Here's how the part is built. I have some questions about the finished solid (model axes, mm). A direction names the side the tool comes from. Coordinates: 2 decimals unless noted, no trailing zeros. Loops run counter-clockwise (first coordinate to the right, second up) from the corner with the lowest first, then second, coordinate; pieces in that order, holes last. Notation, with made-up numbers: M 81,77.5 L 100,77.5 A17 ccw 100,85.5 Z; hole C 71,39 d9. An arc over 180 degrees is marked long. Use CSV: the item, a comma, the result in double quotes. Start each with the question number.
Q1. If we mould it in two halves opening along Z, with no side actions, what happens to faces 3 (the cylindrical face through (103.673, -1.721, 9.021)), 4 (the flat face through (104, 14, 0)), 5 (the cylindrical face through (100.94, 0.8, 5.94))? For each: +Z half, -Z half, draft (parallel to the pull), parting line (faces both ways), or undercut.
Q2. If we section it at C-C (y = 22): Please give me the cut outline in (x, z).
Q3. If we section it at B-B (x = 98.5): Please give me the cut outline in (y, z).
Q4. For pin 1 Ø1.7 at (x, z) = (102.338, 6) entering from +Y, with a flat end and sliding along its axis, tell me the tip position at first contact or that it passes through.
Q5. If we section it at A-A (z = 4): Please give me the cut outline in (x, y), and give its area (3 significant figures).
Q6. Which directions (+Z, -Z, +X, -X, +Y, -Y) give clear straight access to the entire face, cutting with the end or side of a thin tool? Please do faces 1 (the flat face through (101, 10.1, 5)), 2 (the cylindrical face through (100.94, -1.36, 2.29)).
Q7. Please list where these lines run through material, in increasing order: probe 1 along Y at (x, z) = (98.5, 1.25); probe 2 along X at (y, z) = (-0.4, 6); probe 3 along Y at (x, z) = (101.5, 4). Write a range as [from, to].
Autodesk Inventor part; units mm, degrees
ref_plane "YZ Plane" through (0, 0, 0) normal (1, 0, 0) x (0, 1, 0)
ref_plane "XZ Plane" through (0, 0, 0) normal (0, 1, 0) x (-1, 0, 0)
ref_plane "XY Plane" through (0, 0, 0) normal (0, 0, 1) x (1, 0, 0)
ref_plane "Arbeitsebene1" through (0, 0, 0) normal (0, 0, 1) x (1, 0, 0)
sketch "Skizze1" plane through (0, 0, 0) normal (0, 0, 1) x (1, 0, 0)
  line L0 (-118.5, -74.5) -> (-118.5, 74.5)
  arc A0 (-118.5, -74.5) -> (-103.5, -89.5) centre (-103.5, -74.5) ccw
  line L1 (56.1, -89.5) -> (-103.5, -89.5)
  line L2 (56.1, -83) -> (56.1, -89.5)
  arc A1 (71.1, -68) -> (56.1, -83) centre (71.1, -83) ccw
  line L3 (80.5, -68) -> (71.1, -68)
  arc A2 (95.5, -83) -> (80.5, -68) centre (80.5, -83) ccw
  line L4 (95.5, -89.5) -> (95.5, -83)
  line L5 (103.5, -89.5) -> (95.5, -89.5)
  arc A3 (103.5, -89.5) -> (118.5, -74.5) centre (103.5, -74.5) ccw
  line L6 (118.5, 74.5) -> (118.5, -74.5)
  arc A4 (118.5, 74.5) -> (103.5, 89.5) centre (103.5, 74.5) ccw
  line L7 (-103.5, 89.5) -> (103.5, 89.5)
  arc A5 (-103.5, 89.5) -> (-118.5, 74.5) centre (-103.5, 74.5) ccw
  circle A6 centre (-58.5, 18.7) radius 1.4
  circle A7 centre (-58.5, 36.552) radius 1.4
  circle A8 centre (57.5, 20.252) radius 1.4
  circle A9 centre (57.5, 35) radius 1.4
  circle A10 centre (-58.5, 8.7) radius 1.4
  circle A11 centre (-58.5, -9.152) radius 1.4
  circle A12 centre (57.5, 7.148) radius 1.4
  circle A13 centre (57.5, -7.6) radius 1.4
  circle A14 centre (103.5, 74.5) radius 1.4
  circle A15 centre (103.5, -74.5) radius 1.4
  circle A16 centre (-103.5, -74.5) radius 1.4
  circle A17 centre (-103.5, 74.5) radius 1.4
  line L8 (20.9567, 0.5738) -> (-20.9567, 0.5738)
  line L9 (-20.9567, 0.5738) -> (-20.9567, 30.6837)
  line L10 (-20.9567, 30.6837) -> (20.9567, 30.6837)
  line L11 (20.9567, 30.6837) -> (20.9567, 0.5738)
  circle A18 centre (73.1917, -22.4328) radius 1.4
  circle A19 centre (43.1917, -22.4328) radius 1.4
  circle A20 centre (13.1917, -22.4328) radius 1.4
  circle A21 centre (-16.8083, -22.4328) radius 1.4
  circle A22 centre (-46.8083, -22.4328) radius 1.4
  circle A23 centre (-102.338, -1.3) radius 1.4
  circle A24 centre (-102.338, 13.7) radius 1.4
  circle A25 centre (-102.338, 28.7) radius 1.4
  circle A26 centre (102.338, 28.7) radius 1.4
  circle A27 centre (-73.1917, -22.4328) radius 1.4
  circle A28 centre (-43.1917, -22.4328) radius 1.4
  circle A29 centre (-13.1917, -22.4328) radius 1.4
  circle A30 centre (16.8083, -22.4328) radius 1.4
  circle A31 centre (46.8083, -22.4328) radius 1.4
  circle A32 centre (102.338, -1.3) radius 1.4
  circle A33 centre (102.338, 13.7) radius 1.4
  line L12 (97.338, -6.3) -> (107.338, -6.3)
  line L13 (107.338, -6.3) -> (107.338, 33.7)
  line L14 (107.338, 33.7) -> (97.338, 33.7)
  line L15 (97.338, 33.7) -> (97.338, -6.3)
  line L16 (97.338, -6.3) -> (107.338, 33.7) construction
  line L17 (107.338, -6.3) -> (97.338, 33.7) construction
  line L18 (76.5043, -50) -> (76.5043, 50)
  arc A34 (96.5043, 50) -> (76.5043, 50) centre (86.5043, 50) ccw
  line L19 (96.5043, 50) -> (96.5043, -50)
  arc A35 (76.5043, -50) -> (96.5043, -50) centre (86.5043, -50) ccw
  line L20 (-95.8131, -50) -> (-95.8131, 50)
  arc A36 (-75.8131, 50) -> (-95.8131, 50) centre (-85.8131, 50) ccw
  line L21 (-75.8131, 50) -> (-75.8131, -50)
  arc A37 (-95.8131, -50) -> (-75.8131, -50) centre (-85.8131, -50) ccw
  circle A38 centre (-108.5, 79.5) radius 1.4
  circle A39 centre (-108.5, -79.5) radius 1.4
  circle A40 centre (108.5, 79.5) radius 1.4
  circle A41 centre (108.5, -79.5) radius 1.4
  point P0 (0, 0)
  dimension "d0" = 10
  dimension "d1" = 40
extrude "Extrusion1" add sketch "Skizze1" along normal blind 50 contours L15 L14 L13 L12
fillet "Rundung1" radius 5 2 edges at (102.338, -6.3, 50) (102.338, 33.7, 50)
sketch "Skizze2" plane through (97.338, 33.7, 0) normal (0, 1, 0) x (1, 0, 0)
  line L0 (10, -45) -> (0, -45)
  line L1 (10, 0) -> (10, -45)
  line L2 (10, 0) -> (0, 0)
  line L3 (0, 0) -> (0, -45)
  circle A0 centre (5, -6) radius 5
  line L4 (10, 0) -> (10, -45)
  circle A1 centre (5, -6) radius 1.4
  point P0 (-97.338, 0)
  point P1 (0, -6)
  point P2 (10, -6)
  dimension "d5" = 6
  dimension "d8" = 2.8
extrude "Extrusion2" cut sketch "Skizze2" against normal through all contours A0 L3 L2 L1 | A0 keep common part
sketch "Skizze3" plane through (107.338, -6.3, 0) normal (1, 0, 0) x (0, 0, -1)
  line L0 (0, 40) -> (-6, 40)
  line L1 (0, 0) -> (-6, 0)
  line L2 (-4.6, 33.6) -> (0, 33.6)
  line L3 (-4.6, 21.4) -> (0, 21.4)
  line L4 (-4.6, 18.6) -> (0, 18.6)
  line L5 (-4.6, 6.4) -> (0, 6.4)
  line L6 (-4.6, 3.6) -> (0, 3.6)
  line L7 (-4.6, 36.4) -> (0, 36.4)
  line L8 (-11, 40) -> (-11, 0)
  line L9 (-11, 31.6) -> (-1, 31.6)
  line L10 (-1, 31.6) -> (-1, 23.6)
  line L11 (-1, 23.6) -> (-11, 23.6)
  line L12 (-11, 23.6) -> (-11, 31.6)
  line L13 (-11, 16.4) -> (-1, 16.4)
  line L14 (-1, 16.4) -> (-1, 8.4)
  line L15 (-1, 8.4) -> (-11, 8.4)
  line L16 (-11, 8.4) -> (-11, 16.4)
  point P0 (0, 6.3)
  point P1 (-11, 8.4)
  point P2 (-11, 23.6)
  dimension "d9" = 10
  dimension "d10" = 8
  dimension "d11" = 10
  dimension "d12" = 8
  dimension "d13" = 2
  dimension "d14" = 2.2
extrude "Extrusion3" cut sketch "Skizze3" against normal blind 10
properties part number "60_Planktoscope_Illuminationsource"
Results below:
1,face 3,"draft"
1,face 4,"-Z half"
1,face 5,"undercut"
2,outline,"M 97.34,0 L 107.34,0 L 107.34,1 L 97.34,1 Z"
3,outline,"M -6.3,0 L 33.7,0 L 33.7,9.2 L 25.3,9.2 L 25.3,1 L 17.3,1 L 17.3,9.2 L 10.1,9.2 L 10.1,1 L 2.1,1 L 2.1,9.2 L -6.3,9.2 Z"
4,pin 1,"through"
5,outline,"M 97.34,-6.3 L 107.34,-6.3 L 107.34,2.1 L 97.34,2.1 Z; M 97.34,10.1 L 107.34,10.1 L 107.34,17.3 L 97.34,17.3 Z; M 97.34,25.3 L 107.34,25.3 L 107.34,33.7 L 97.34,33.7 Z; hole C 102.34,-1.3 d2.8; hole C 102.34,13.7 d2.8; hole C 102.34,28.7 d2.8"
5,area,"222 mm^2"
6,face 1,"+Z, +X, -X"
6,face 2,"+Z, -Z"
7,probe 1,"[-6.3, 2.1], [10.1, 17.3], [25.3, 33.7]"
7,probe 2,"[97.34, 100.94], [103.74, 107.34]"
7,probe 3,"[-6.3, -2.42], [-0.18, 2.1], [10.1, 12.58], [14.82, 17.3], [25.3, 27.58], [29.82, 33.7]"
